Geometry check sheet. Reference: drawing and pictorial views, mm from the part's lowest x, y, z. A direction names the side the tool comes from. Coordinates: 2 decimals unless noted, no trailing zeros. Write each loop counter-clockwise with the first axis right and the second up, starting at its lowest first coordinate (ties: lowest second). Pieces come first, ordered by that corner, then holes. Notation, with made-up numbers: (56, 59) -> (71, 59) arc R14 ccw to (71, 68) -> close; hole circle Ø6 at (13.25, -21.75). An arc over 180 degrees is marked (long way). Use a Markdown table: item, result.
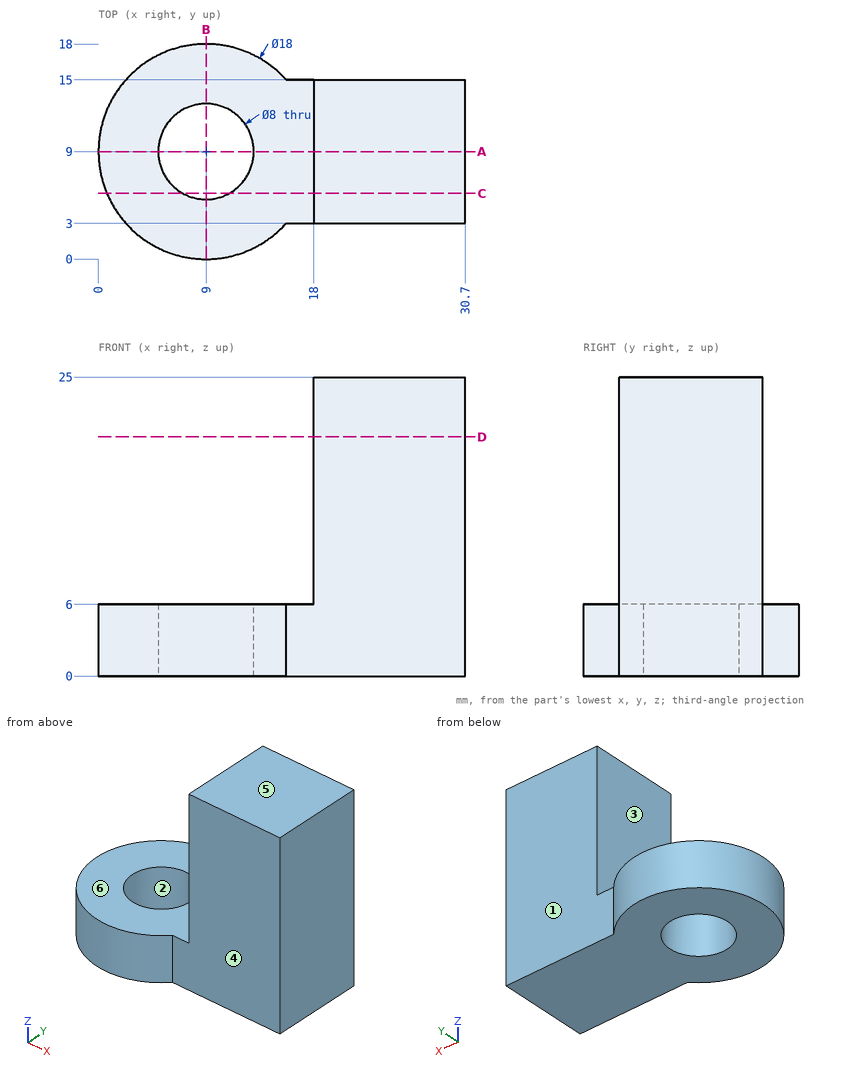
Item 1: Depth check by flat-ended pin: P1, Ø12, axis at x = 20, z = 16, coming from the -Y side; P2, Ø1, axis at y = 12, z = 4.5, coming from the -X side; P3, Ø6, axis at x = 18, y = 11.5, coming from the -Z side; P4, Ø10, axis at y = 9.5, z = 14.5, coming from the -X side. Enter the tip coordinate at first touch or a pass-through.
Answer block:
| item | result |
|---|---|
| P1 | stops at y = 3 |
| P2 | stops at x = 0.35 |
| P3 | stops at z = 0 |
| P4 | stops at x = 18 |
Item 2: Tool access check on the marked faces 4, 5 and 6. Record the directions out of +Z, -Z, +X, -X, +Y, -Y that give a thin tool (end or side, any length) a straight path to the whole face; none if there is none.
Answer block:
| item | result |
|---|---|
| face 4 | +Z, -Z, +X, -Y |
| face 5 | +Z, +X, -X, +Y, -Y |
| face 6 | +Z, -X, +Y, -Y |
Item 3: Mould release check, pull along X, two halves, no side actions. Record for the marked faces 1, 2 and 3: +X half, -X half, draft (parallel to the pull), parting line (faces both ways), or undercut.
Answer block:
| item | result |
|---|---|
| face 1 | draft |
| face 2 | undercut |
| face 3 | -X half |
Item 4: Section check A-A on y = 9. Record the boundary of the cut face in (x, z), then the cut area to 4 significant figures.
Answer block:
| item | result |
|---|---|
| outline | (0, 0) -> (5, 0) -> (5, 6) -> (0, 6) -> close; (13, 0) -> (30.7, 0) -> (30.7, 25) -> (18, 25) -> (18, 6) -> (13, 6) -> close |
| area | 377.5 mm^2 |
Item 5: Section check D-D on z = 20. Record the boundary of the cut face in (x, y), then the cut area to 3 significant figures.
Answer block:
| item | result |
|---|---|
| outline | (18, 3) -> (30.7, 3) -> (30.7, 15) -> (18, 15) -> close |
| area | 152 mm^2 |
Item 6: Section check B-B on x = 9. Record the boundary of the cut face in (y, z), then the cut area to 3 significant figures.
Answer block:
| item | result |
|---|---|
| outline | (0, 0) -> (5, 0) -> (5, 6) -> (0, 6) -> close; (13, 0) -> (18, 0) -> (18, 6) -> (13, 6) -> close |
| area | 60.0 mm^2 |
Item 7: Section check C-C on y = 5.5. Record the boundary of the cut face in (x, z).
Answer block:
| item | result |
|---|---|
| outline | (0.71, 0) -> (7.06, 0) -> (7.06, 6) -> (0.71, 6) -> close; (10.94, 0) -> (30.7, 0) -> (30.7, 25) -> (18, 25) -> (18, 6) -> (10.94, 6) -> close |
Item 8: Thickness scan on L1, parallel to Y at x = 9, z = 1.7; L2, parallel to Z at x = 7, y = 2; L3, parallel to X at y = 10.75, z = 14.5. Record the ranges inside material, lowest first. Write a range as [from, to].
Answer block:
| item | result |
|---|---|
| L1 | y = [0, 5], [13, 18] |
| L2 | z = [0, 6] |
| L3 | x = [18, 30.7] |
